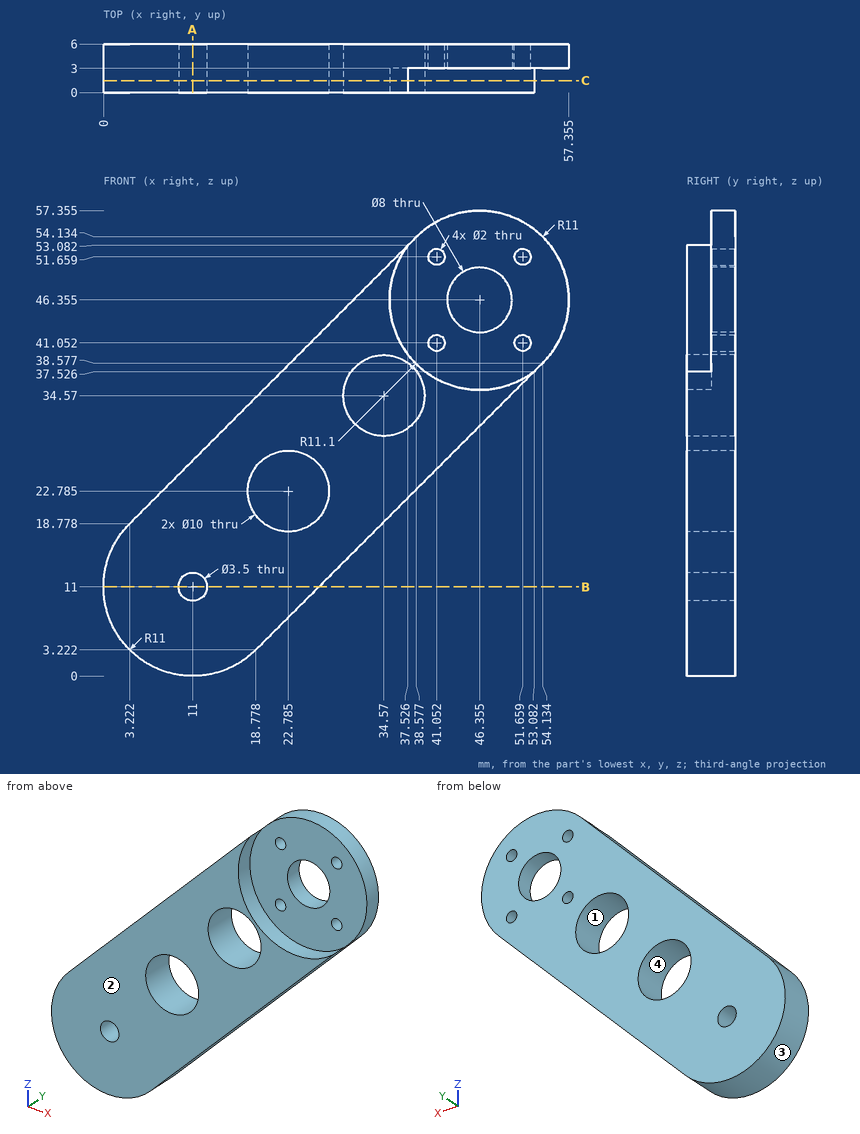
Geometry: see drawing. Coordinates: mm, zero at the bounding-box minimum. Give positions to 0.01 mm unless a question says otherwise; leave off trailing zeros. Loops run counter-clockwise (first coordinate to the right, second up) from the corner with the lowest first, then second, coordinate; pieces in that order, holes last. Notation, with made-up numbers: (62, 72) -> (107, 72) arc R9 ccw to (107, 80) -> close; hole circle Ø8 at (-10.75, -23). An arc over 180 degrees is marked (long way). Use CSV: the item, a comma, the result in double quotes.
(1) Cut plane B-B (z = 11). Output: boundary loops of the cut face in (x, y).
From the geometry:
outline,"(0, 0) -> (9.25, 0) -> (9.25, 6) -> (0, 6) -> close; (12.75, 0) -> (26.56, 0) -> (26.56, 6) -> (12.75, 6) -> close"
(2) Ray query, line 1 along Y through (x, z) = (38.5, 41); line 2 along X through (y, z) = (4.25, 44) (1 decimal); line 3 along X through (y, z) = (3.75, 30.5) (1 decimal). Return the intervals inside material, ascending. Write a range as [from, to].
From the geometry:
line 1,"[3, 6]"
line 2,"[28.4, 43.1], [49.6, 57.1]"
line 3,"[14.9, 31.7], [37.5, 46.1]"
(3) Pull-direction query (X, two-part tool) for the marked faces 1, 2, 3 and 4; classes: released by +X, released by -X, zero draft, split by the parting line, or undercut.
From the geometry:
face 1,"undercut"
face 2,"zero draft"
face 3,"split by the parting line"
face 4,"undercut"
(4) First-contact query: P1, Ø2, axis at y = 5, z = 19.5, coming from the +X side (1 decimal); P2, Ø3, axis at x = 51.66, z = 51.66, coming from the -Y side; P3, Ø3, axis at y = 2, z = 42, coming from the +X side. Flat tips, straight axial feed; report the tip coordinate or a pass-through.
From the geometry:
P1,"x = 36.1"
P2,"y = 3"
P3,"x = 56.87"
(5) Cut plane C-C (y = 1.5). Count the separate pieces of the cut face and the enclosed holes in it, plus the area to 3 significant figures.
From the geometry:
separate pieces,"1"
enclosed holes,"3"
area,"930 mm^2"
(6) Cut plane A-A (x = 11). Output: boundary loops of the cut face in (y, z).
From the geometry:
outline,"(0, 0) -> (6, 0) -> (6, 9.25) -> (0, 9.25) -> close; (0, 12.75) -> (6, 12.75) -> (6, 26.56) -> (0, 26.56) -> close"
